from build123d import *

# Parameters (mm, degrees)
F0_W     = 46.001066
F0_H     = 45.813687
F1_DEPTH = 25.4
F2_R     = 5.772308
F3_DEPTH = 46.002066


with BuildPart() as f1:
    # F0 (on Front) → F1 (new body)
    with BuildSketch(Plane.XZ):
        with Locations((23.000533, 22.906843)):
            Rectangle(F0_W, F0_H)
    extrude(amount=F1_DEPTH)

    # F2 (on Right) → F3 (cut, through all)
    with BuildSketch(Plane.YZ):
        with Locations((-16.395491, 29.137131)):
            Circle(F2_R)
    extrude(amount=F3_DEPTH, mode=Mode.SUBTRACT)


solid = f1.part
Can you work these out from the model? Positions are in its coordinate system, mm. Coordinates: 2 decimals unless noted, no trailing zeros. Write each loop counter-clockwise with the first axis right and the second up, starting at its lowest first coordinate (ties: lowest second). Pieces come first, ordered by that corner, then holes. Notation, with made-up numbers: (69, -20.75) -> (103, -20.75) arc R3 cw to (103, -15.75) -> close; hole circle Ø9 at (64, -31). An arc over 180 degrees is marked (long way). Write item = value, one per line.
(1) Imagine slicing it at C-C (x = 30.5). Please give me the cut outline in (y, z).
Verdict:
outline = (-25.4, 0) -> (0, 0) -> (0, 45.81) -> (-25.4, 45.81) -> close; hole circle Ø11.54 at (-16.4, 29.14)
(2) Imagine slicing it at B-B (z = 33). Please give me the cut outline in (x, y), and give its area (3 significant figures).
Verdict:
outline = (0, -25.4) -> (46, -25.4) -> (46, -20.68) -> (0, -20.68) -> close; (0, -12.11) -> (46, -12.11) -> (46, 0) -> (0, 0) -> close
area = 774 mm^2
(3) Thinking about a two-plate mould opening in Z: for faces 1 (the face through (46.001, -13, 23)), 2 (the face through (23, -13, 0)), 3 (the face through (22.679, -22.162, 29.391)), which applies, +Z half, -Z half, draft (parallel to the pull), parting line (faces both ways), or undercut?
Verdict:
face_1 = draft
face_2 = -Z half
face_3 = undercut
(4) Imagine slicing it at A-A (y = -18.75). Please give me the cut outline in (x, z).
Verdict:
outline = (0, 0) -> (46, 0) -> (46, 23.87) -> (0, 23.87) -> close; (0, 34.41) -> (46, 34.41) -> (46, 45.81) -> (0, 45.81) -> close
(5) If I drill on probe 1 along Y at (x, z) = (41, 29); probe 2 along Y at (x, z) = (31, 26); probe 3 along Z at (x, y) = (43.5, -14.5), over which ranges is the centre line in solid material (lowest first)?
Verdict:
probe_1 = -25.4 to -22.17, -10.62 to 0
probe_2 = -25.4 to -21.24, -11.55 to 0
probe_3 = 0 to 23.68, 34.59 to 45.81
